Part print with two shaded views. Sizes in mm from the minimum x, y, z corner. Coordinates: 2 decimals unless noted, no trailing zeros. Loops run counter-clockwise (first coordinate to the right, second up) from the corner with the lowest first, then second, coordinate; pieces in that order, holes last.
Item 1: Cut at A-A (x = 12). List the corners of the cut face in (y, z), and give its area (3 significant figures).
Item 2: Cut at B-B (z = 10.5). List the corners of the cut face in (x, y).
Item 3: Cut at D-D (z = 1). List the corners of the cut face in (x, y), and give its area (3 significant figures).
Item 4: Cut at C-C (y = 16.75). List the corners of the cut face in (x, z).
Item 5: Mould opens along X. For the marked faces 1, 2 and 3 say: released by +X, released by -X, zero draft, split by the parting line, or undercut.
Item 6: Flat gauge pin, fed straight in: pin 1 (3 mm diameter, centred on x = 19, z = 10.5, fed in from +Y). Where does the tip first touch, or does it go through?
Item 7: Drill centre lines: line 1 along X through (y, z) = (5.5, 11); line 2 along X through (y, z) = (14.75, 8.75); line 3 along Z through (x, y) = (12, 12.75). Where is each one in solid material? Low to high.
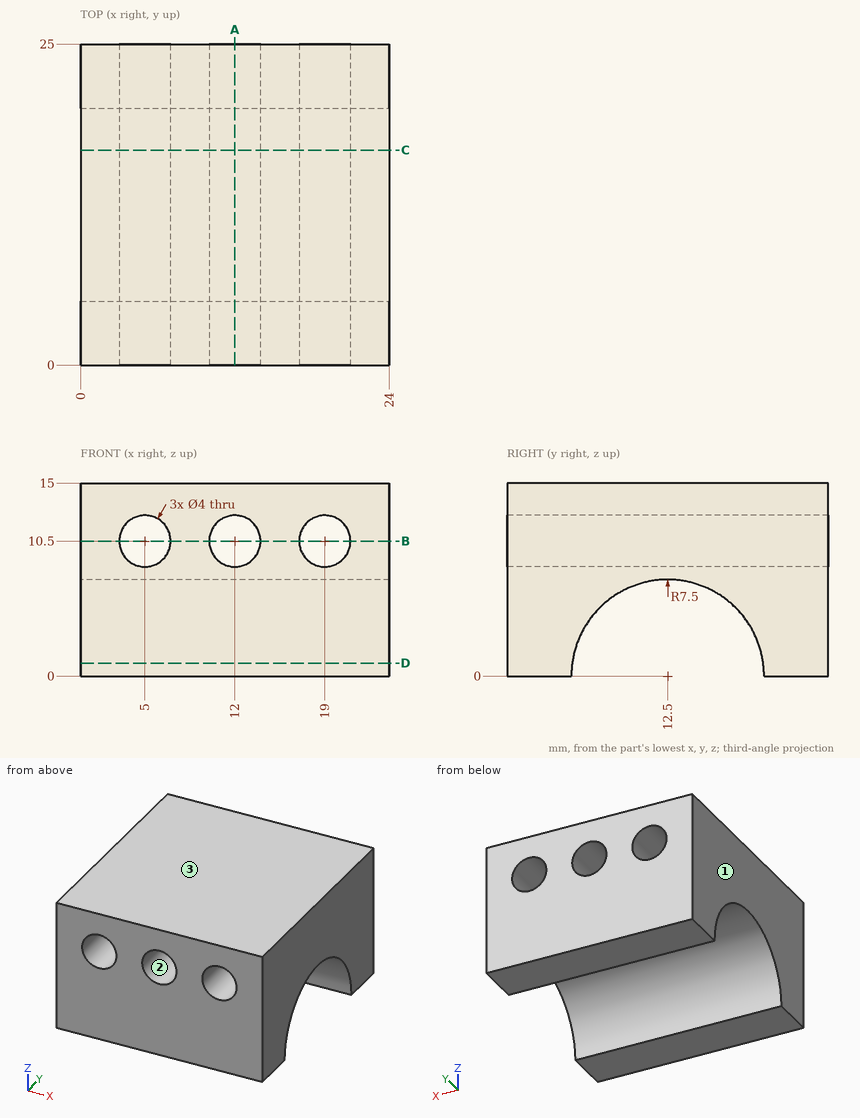
Filled sheet:
1. outline: (0, 0) - (5, 0) arc R7.5 cw to (20, 0) - (25, 0) - (25, 8.5) - (0, 8.5) - close; (0, 12.5) - (25, 12.5) - (25, 15) - (0, 15) - close
1. area: 187 mm2
2. outline: (0, 0) - (3, 0) - (3, 25) - (0, 25) - close; (7, 0) - (10, 0) - (10, 25) - (7, 25) - close; (14, 0) - (17, 0) - (17, 25) - (14, 25) - close; (21, 0) - (24, 0) - (24, 25) - (21, 25) - close
3. outline: (0, 0) - (24, 0) - (24, 5.07) - (0, 5.07) - close; (0, 19.93) - (24, 19.93) - (24, 25) - (0, 25) - close
3. area: 243 mm2
4. outline: (0, 6.18) - (24, 6.18) - (24, 15) - (0, 15) - close; hole circle Ø4 at (5, 10.5); hole circle Ø4 at (12, 10.5); hole circle Ø4 at (19, 10.5)
5. face 1: released by -X
5. face 2: undercut
5. face 3: zero draft
6. pin 1: passes through
7. line 1: x = 0 to 3.06, 6.94 to 10.06, 13.94 to 17.06, 20.94 to 24
7. line 2: x = 0 to 4.03, 5.97 to 11.03, 12.97 to 18.03, 19.97 to 24
7. line 3: z = 7.5 to 8.5, 12.5 to 15
